The drawing under review shows one solid part. Ordinate dimensions are in mm from its lowest x, y, z. Coordinates: 2 decimals unless noted, no trailing zeros. Order: outer loops, then holes, each group sorted by start corner. A loop starts at its lowest first (then second) coordinate and runs counter-clockwise, first axis right, second up.
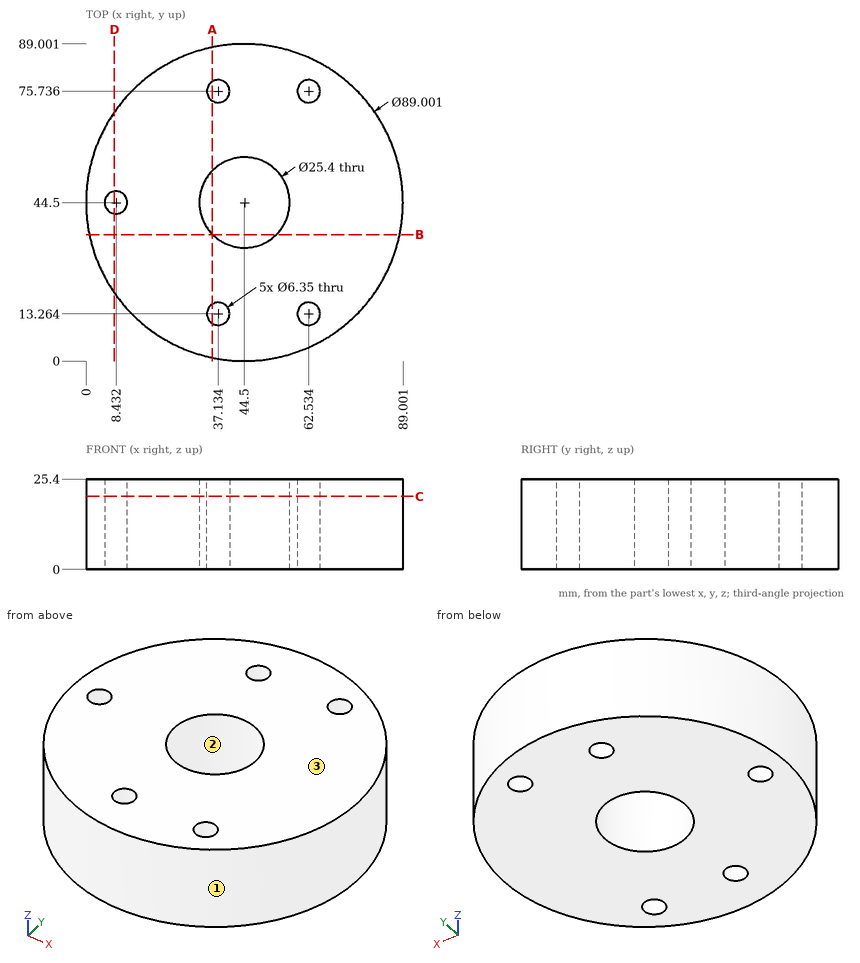
(1) Wall thickness on probe 1 along Y at (x, z) = (45, 5.5); probe 2 along Y at (x, z) = (11, 23.5) (1 decimal); probe 3 along Y at (x, z) = (62.5, 23): over which ranges is each line inside the solid? List them lowest first.
A:
probe 1: y = 0 to 31.81, 57.19 to 89
probe 2: y = 15.2 to 42.6, 46.4 to 73.8
probe 3: y = 3.8 to 10.09, 16.44 to 72.56, 78.91 to 85.2
(2) Draft analysis for pull direction Y (two halves, no side actions). For the marked faces 1, 2 and 3, state which applies: released by +Y, released by -Y, zero draft, split by the parting line, or undercut.
A:
face 1: split by the parting line
face 2: undercut
face 3: zero draft
(3) We need section C-C, the plane z = 20.5. Count the separate pieces of the cut face and the enclosed holes in it, and give its area (3 significant figures).
A:
separate pieces: 1
enclosed holes: 6
area: 5,560 mm2
(4) We need section A-A, the plane x = 35.5. Write out the cut boundary in (y, z), and give its area (3 significant figures).
A:
outline: (0.92, 0) - (10.54, 0) - (10.54, 25.4) - (0.92, 25.4) - close; (15.99, 0) - (35.54, 0) - (35.54, 25.4) - (15.99, 25.4) - close; (53.46, 0) - (73.01, 0) - (73.01, 25.4) - (53.46, 25.4) - close; (78.46, 0) - (88.08, 0) - (88.08, 25.4) - (78.46, 25.4) - close
area: 1,480 mm2
(5) For pin 1 Ø8.5 at (x, y) = (37.13, 13.26) entering from +Z; pin 2 Ø2 at (x, z) = (58, 13) entering from +Y; pin 3 Ø8 at (y, z) = (74.5, 16.5) entering from +X (1 decimal); pin 4 Ø2 at (x, z) = (33.5, 20) entering from -Y, all flat-tipped, find the tip position at first contact; note any pin that passes through.
A:
pin 1: stops at z = 25.4
pin 2: stops at y = 87.21
pin 3: stops at x = 80.6
pin 4: stops at y = 1.14
(6) We need section D-D, the plane x = 8. Write out the cut boundary in (y, z) (1 decimal).
A:
outline: (19, 0) - (41.4, 0) - (41.4, 25.4) - (19, 25.4) - close; (47.6, 0) - (70, 0) - (70, 25.4) - (47.6, 25.4) - close
(7) We need section B-B, the plane y = 35.5. Write out the cut boundary in (x, z).
A:
outline: (0.92, 0) - (35.54, 0) - (35.54, 25.4) - (0.92, 25.4) - close; (53.46, 0) - (88.08, 0) - (88.08, 25.4) - (53.46, 25.4) - close
